```python
from build123d import *

# Parameters (mm, degrees)
ESQUISSE1_R        = 1.5
ESQUISSE1_R_2      = 2.5
ESQUISSE1_W        = 5
ESQUISSE1_H        = 5
BOSS_EXTRU_1_DEPTH = 5


with BuildPart() as part:
    # Esquisse1 → Boss.-Extru.1 (new body)
    with BuildSketch(Plane.XY):
        with BuildLine():
            Line((8, 0), (39, 0))
            ThreePointArc((39, 0), (44.656854249, 2.343145751), (47, 8))
            Line((47, 8), (47, 22))
            ThreePointArc((47, 22), (44.656854249, 27.656854249), (39, 30))
            Line((39, 30), (8, 30))
            ThreePointArc((8, 30), (2.343145751, 27.656854249), (0, 22))
            Line((0, 22), (0, 8))
            ThreePointArc((0, 8), (2.343145751, 2.343145751), (8, 0))
        make_face()
        with Locations((7.5, 15)):
            Circle(ESQUISSE1_R, mode=Mode.SUBTRACT)
        with Locations((39.5, 15)):
            Circle(ESQUISSE1_R, mode=Mode.SUBTRACT)
        with Locations((23.5, 15)):
            Circle(ESQUISSE1_R_2, mode=Mode.SUBTRACT)
        with Locations((7.5, 22.5)):
            Rectangle(ESQUISSE1_W, ESQUISSE1_H, mode=Mode.SUBTRACT)
        with Locations((39.5, 22.5)):
            Rectangle(ESQUISSE1_W, ESQUISSE1_H, mode=Mode.SUBTRACT)
        with Locations((39.5, 7.5)):
            Rectangle(ESQUISSE1_W, ESQUISSE1_H, mode=Mode.SUBTRACT)
        with Locations((7.5, 7.5)):
            Rectangle(ESQUISSE1_W, ESQUISSE1_H, mode=Mode.SUBTRACT)
    extrude(amount=BOSS_EXTRU_1_DEPTH)


solid = part.part
```
Source: CAD feature listing. Evaluate the final solid. Frame: model axes, mm. A direction names the side the tool comes from. Give positions to 0.01 mm unless a question says otherwise; leave off trailing zeros. Write each loop counter-clockwise with the first axis right and the second up, starting at its lowest first coordinate (ties: lowest second). Pieces come first, ordered by that corner, then holes.
1. Material intervals for line 1 along X through (y, z) = (22, 3.8); line 2 along X through (y, z) = (23, 2.4); line 3 along X through (y, z) = (14, 1.95), sorted ascending.
2. First-contact query: pin 1 (1.5 mm diameter, centred on y = 22.5, z = 2.5, fed in from +X); pin 2 (1.5 mm diameter, centred on y = 4.5, z = 3.5, fed in from +X). Flat tips, straight axial feed; report the tip coordinate or a pass-through.
3. Section query C-C (y = 15). Return the cut outline in (x, z), then the cut area to 3 significant figures.
4. Section query D-D (x = 23.5). Return the cut outline in (y, z).
5. Section query B-B (z = 2.55). Return the cut outline in (x, y), then the cut area to 3 significant figures.
6. Pull-direction query (X, two-part tool) for faces 3 (the face through (23, 0, 2)), 4 (the face through (39, 20, 2)), 5 (the face through (2.406, 27.719, 2.465)); classes: +X half, -X half, draft (parallel to the pull), parting line (faces both ways), or undercut.
7. Section query A-A (y = 8.5). Return the cut outline in (x, z).
8. Access query for faces 1 (the face through (42, 22, 2)), 2 (the face through (47, 15, 2)). Directions: +Z, -Z, +X, -X, +Y, -Y. A direction counts if a zero-diameter tool reaches every point of the face in a straight line with its end or side. Return the directions, or none.
Output values:
1. line 1: x = 0 to 5, 10 to 37, 42 to 47
1. line 2: x = 0.06 to 5, 10 to 37, 42 to 46.94
1. line 3: x = 0 to 6.38, 8.62 to 21.21, 25.79 to 38.38, 40.62 to 47
2. pin 1: stops at x = 47
2. pin 2: stops at x = 46.51
3. outline: (0, 0) - (6, 0) - (6, 5) - (0, 5) - close; (9, 0) - (21, 0) - (21, 5) - (9, 5) - close; (26, 0) - (38, 0) - (38, 5) - (26, 5) - close; (41, 0) - (47, 0) - (47, 5) - (41, 5) - close
3. area: 180 mm2
4. outline: (0, 0) - (12.5, 0) - (12.5, 5) - (0, 5) - close; (17.5, 0) - (30, 0) - (30, 5) - (17.5, 5) - close
5. outline: (0, 8) arc R8 ccw to (8, 0) - (39, 0) arc R8 ccw to (47, 8) - (47, 22) arc R8 ccw to (39, 30) - (8, 30) arc R8 ccw to (0, 22) - close; hole (5, 5) - (10, 5) - (10, 10) - (5, 10) - close; hole (5, 20) - (10, 20) - (10, 25) - (5, 25) - close; hole circle Ø3 at (7.5, 15); hole circle Ø5 at (23.5, 15); hole (37, 5) - (42, 5) - (42, 10) - (37, 10) - close; hole (37, 20) - (42, 20) - (42, 25) - (37, 25) - close; hole circle Ø3 at (39.5, 15)
5. area: 1,220 mm2
6. face 3: draft
6. face 4: undercut
6. face 5: -X half
7. outline: (0, 0) - (5, 0) - (5, 5) - (0, 5) - close; (10, 0) - (37, 0) - (37, 5) - (10, 5) - close; (42, 0) - (47, 0) - (47, 5) - (42, 5) - close
8. face 1: +Z, -Z
8. face 2: +Z, -Z, +X, +Y, -Y
